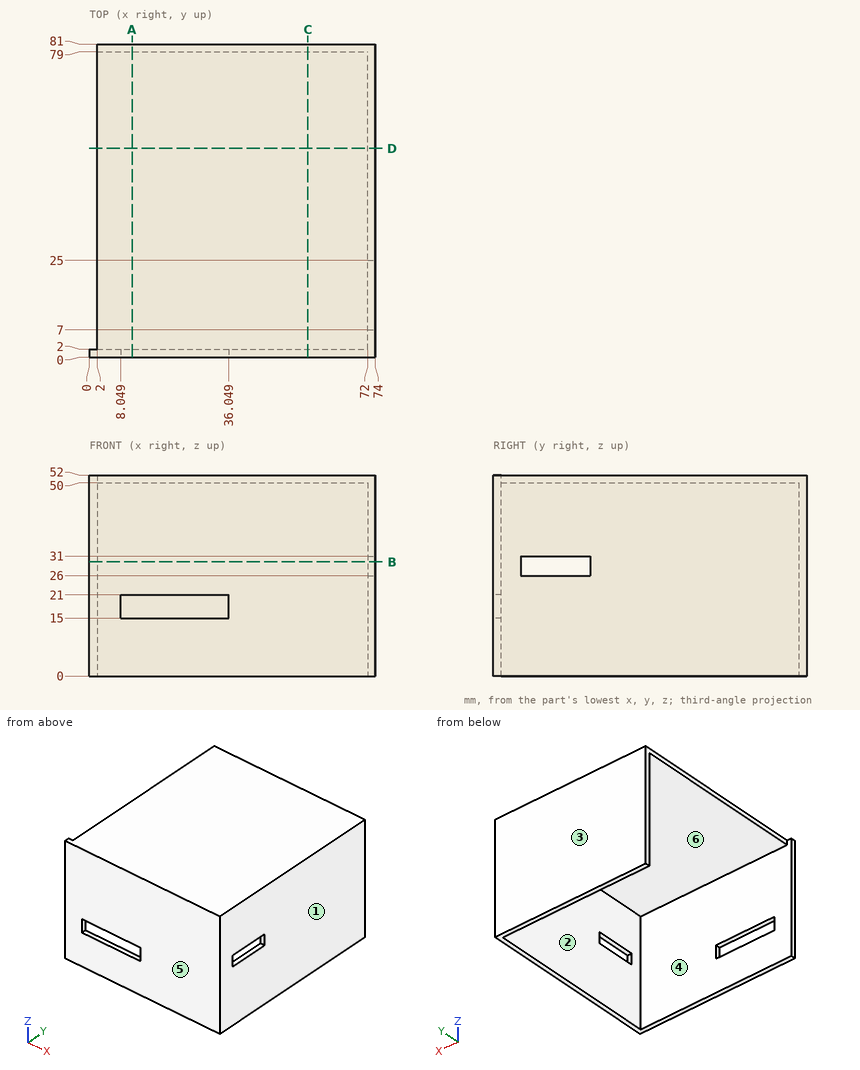
Could you check a few things on this drawing? It's one solid part, dimensions in mm from its lowest x, y, z. A direction names the side the tool comes from. Coordinates: 2 decimals unless noted, no trailing zeros. Write each loop counter-clockwise with the first axis right and the second up, starting at its lowest first coordinate (ties: lowest second). Pieces come first, ordered by that corner, then holes. Notation, with made-up numbers: (72, 36) - (98, 36) arc R28 cw to (98, 64) - close; hole circle Ø1 at (41.5, -19). An arc over 180 degrees is marked (long way). Put each result on its own line as item: value. Start each with the question number.
Q1. Thinking about a two-plate mould opening in Y: for the marked faces 1, 2, 3 and 4, which applies, pulls with the +Y half, pulls with the -Y half, needs draft (parallel to the pull), parting line crosses it, or undercut?
Q2. I want a section at B-B on z = 29.5. Write out the boundary of the cut face in (x, y).
Q3. I want a section at D-D on y = 54. Write out the boundary of the cut face in (x, z).
Q4. Please list where these lines run through material, in increasing order: L1, parallel to Y at x = 49, z = 21; L2, parallel to X at y = 4.5, z = 47.5; L3, parallel to Z at x = 32, y = 24.5.
Q5. I want a section at C-C on x = 56.5. Write out the boundary of the cut face in (y, z).
Q6. I'm going to push flat-ended pins straight in: P1, Ø1.5, axis at y = 55, z = 8.5, coming from the -X side; P2, Ø2, axis at x = 57, y = 18.5, coming from the -Z side. Where does each tip first touch, or does it pass through?
Q7. Which directions (+Z, -Z, +X, -X, +Y, -Y) give clear straight access to the entire face, cutting with the end or side of a thin tool? Please do the marked faces 5 and 6.
Q8. I want a section at A-A on x = 11. Write out the boundary of the cut face in (y, z).
Checks:
1. face 1: needs draft
1. face 2: undercut
1. face 3: pulls with the +Y half
1. face 4: undercut
2. outline: (0, 0) - (74, 0) - (74, 7) - (72, 7) - (72, 2) - (0, 2) - close; (2, 79) - (72, 79) - (72, 25) - (74, 25) - (74, 81) - (2, 81) - close
3. outline: (2, 50) - (72, 50) - (72, 0) - (74, 0) - (74, 52) - (2, 52) - close
4. L1: 0 to 2, 79 to 81
4. L2: 72 to 74
4. L3: 50 to 52
5. outline: (0, 0) - (2, 0) - (2, 50) - (79, 50) - (79, 0) - (81, 0) - (81, 52) - (0, 52) - close
6. P1: x = 72
6. P2: z = 50
7. face 5: +Z, -Z, +X, -X, -Y
7. face 6: -Z, -X
8. outline: (0, 0) - (2, 0) - (2, 15) - (0, 15) - close; (0, 21) - (2, 21) - (2, 50) - (79, 50) - (79, 0) - (81, 0) - (81, 52) - (0, 52) - close
